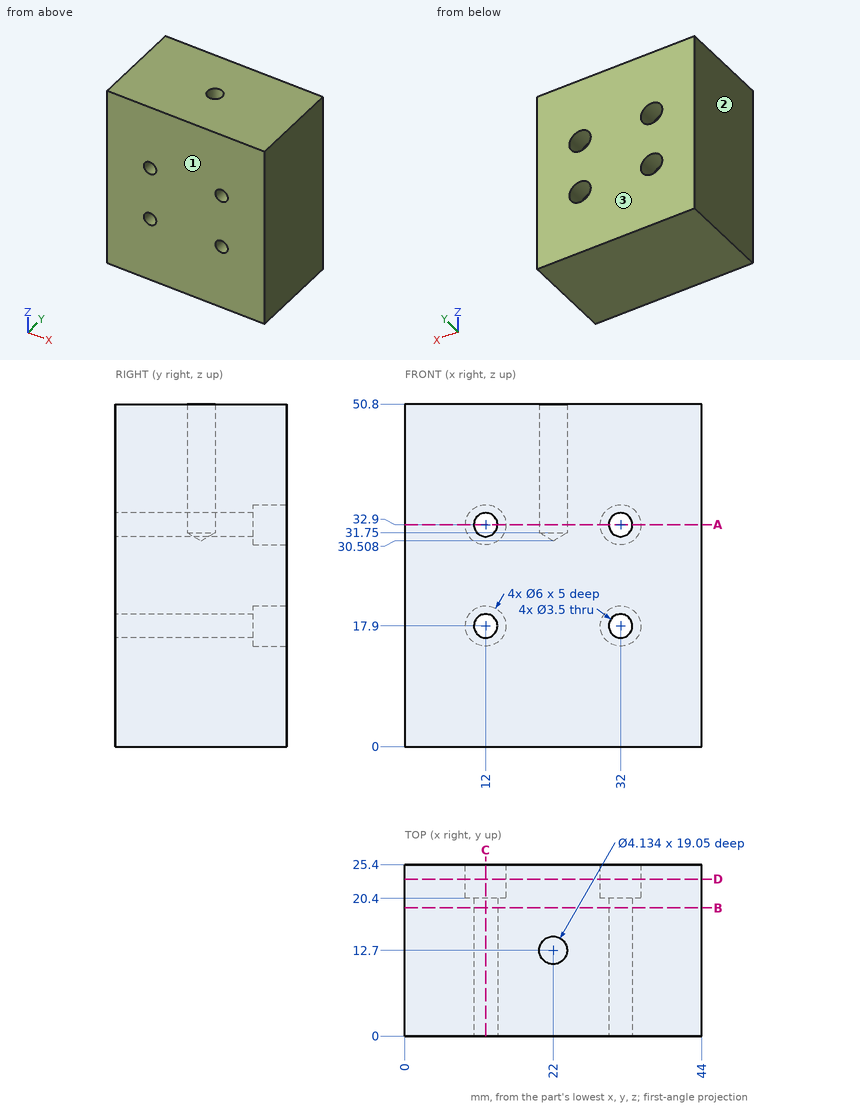
The figure shows three views and two pictorial views of one solid part (mm, origin at its lowest corner). Answer the questions. Give positions to 0.01 mm unless a question says otherwise; leave off trailing zeros. Order: outer loops, then holes, each group sorted by start corner. A loop starts at its lowest first (then second) coordinate and runs counter-clockwise, first axis right, second up. Notation, with made-up numbers: M -9.75,79.25 L 23.25,79.25 A8 cw 23.25,85.25 Z; hole C 36.5,42 d10. An arc over 180 degrees is marked long. Return JSON: item names as keys, results as strings.
Q1. Find the intervals of material crossed by line 1 along X through (y, z) = (4.5, 18); line 2 along Z through (x, y) = (12, 10.5); line 3 along Z through (x, y) = (33.5, 6.5), in increasing order. Write a range as [from, to].
Answer below:
{"line 1": "x = [0, 10.25], [13.75, 30.25], [33.75, 44]", "line 2": "z = [0, 16.15], [19.65, 31.15], [34.65, 50.8]", "line 3": "z = [0, 17], [18.8, 32], [33.8, 50.8]"}
Q2. Find section A-A, the plane z = 32.9. Write down the section's boundary in (x, y).
Answer below:
{"outline": "M 0,0 L 10.25,0 L 10.25,20.4 L 9,20.4 L 9,25.4 L 0,25.4 Z; M 13.75,0 L 30.25,0 L 30.25,20.4 L 29,20.4 L 29,25.4 L 15,25.4 L 15,20.4 L 13.75,20.4 Z; M 33.75,0 L 44,0 L 44,25.4 L 35,25.4 L 35,20.4 L 33.75,20.4 Z; hole C 22,12.7 d4.13"}
Q3. Find section B-B, the plane y = 19. Write down the section's boundary in (x, z), and give its area (3 significant figures).
Answer below:
{"outline": "M 0,0 L 44,0 L 44,50.8 L 0,50.8 Z; hole C 12,17.9 d3.5; hole C 12,32.9 d3.5; hole C 32,17.9 d3.5; hole C 32,32.9 d3.5", "area": "2,200 mm^2"}
Q4. Find section D-D, the plane y = 23.25. Write down the section's boundary in (x, z).
Answer below:
{"outline": "M 0,0 L 44,0 L 44,50.8 L 0,50.8 Z; hole C 12,17.9 d6; hole C 12,32.9 d6; hole C 32,17.9 d6; hole C 32,32.9 d6"}
Q5. Find section C-C, the plane x = 12. Write down the section's boundary in (y, z), and give its area (3 significant figures).
Answer below:
{"outline": "M 0,0 L 25.4,0 L 25.4,14.9 L 20.4,14.9 L 20.4,16.15 L 0,16.15 Z; M 0,19.65 L 20.4,19.65 L 20.4,20.9 L 25.4,20.9 L 25.4,29.9 L 20.4,29.9 L 20.4,31.15 L 0,31.15 Z; M 0,34.65 L 20.4,34.65 L 20.4,35.9 L 25.4,35.9 L 25.4,50.8 L 0,50.8 Z", "area": "1,090 mm^2"}
Q6. The mould has two halves that part along Y. Classify the marked faces 1, 2 and 3: pulls with the +Y half, pulls with the -Y half, needs draft (parallel to the pull), parting line crosses it, or undercut.
Answer below:
{"face 1": "pulls with the -Y half", "face 2": "needs draft", "face 3": "pulls with the +Y half"}
Q7. Each of these flat-tipped pins is pushed along its axis until it touches: pin 1 (2 mm diameter, centred on x = 30, z = 29, fed in from -Y); pin 2 (3 mm diameter, centred on x = 11.5, z = 19, fed in from +Y); pin 3 (3 mm diameter, centred on x = 32, z = 17.9, fed in from +Y). Where does it stop, or does it pass through?
Answer below:
{"pin 1": "stops at y = 0", "pin 2": "stops at y = 20.4", "pin 3": "passes through"}
